The model under review builds one solid part; all positions refer to its coordinate system, in mm. A direction names the side the tool comes from. Coordinates: 2 decimals unless noted, no trailing zeros. Write each loop counter-clockwise with the first axis right and the second up, starting at its lowest first coordinate (ties: lowest second). Pieces come first, ordered by that corner, then holes.
1) For line 1 (Y direction, x = -28, z = 9); line 2 (X direction, y = -11.5, z = 5.5); line 3 (X direction, y = -22.5, z = 9.5), list the stretches that pass through material, from the lowest coordinate up.
2) Add section C-C, the plane y = -21. State the section outline as (x, z) points, then the cut area to 3 significant figures.
3) Add section A-A, the plane z = 6. State the section outline as (x, y) points.
4) For P1, Ø3, axis at y = 9, z = 7.5, coming from the +X side; P2, Ø2, axis at x = -16, y = 25.5, coming from the +Z side; P3, Ø5, axis at x = 2.5, z = 5, coming from the +Y side; P4, Ø1, axis at x = -36.5, z = 4, coming from the -Y side, all flat-tipped, find the tip position at first contact; note any pin that passes through.
5) Add section B-B, the plane x = 32. State the section outline as (y, z) points, then the cut area to 3 significant figures.
6) Mouldability with a two-part tool opening along Y and no side actions: class faces 1 (the conical face through (36.221, -23.091, 11.017)), 2 (the flat face through (0, -25.15, 7)), 3 (the flat face through (-39.3, 0.3, 2)) as released by +Y, released by -Y, zero draft, split by the parting line, or undercut.
7) Machinability: for faces 4 (the flat face through (-38.3, 0, 7)), 5 (the conical face through (-36.221, 23.091, 11.017)), 6 (the flat face through (36.3, 0, 6)), 7 (the cylindrical face through (-37.4, -24.29, 7.19)), 8 (the flat face through (0, 25.15, 7)), which of the approach directions +Z, -Z, +X, -X, +Y, -Y give a long, thin tool a straight path to every point of the face, cutting with its end or side? Answer none if there is none.
Autodesk Fusion 360 part; units mm, degrees
sketch "Sketch1" plane through (0, 0, 0) normal (0, 0, 1) x (1, 0, 0)
  line L0 (36, -22.85) -> (-36, -22.85) construction
  line L1 (-36, -22.85) -> (-36, 22.85) construction
  line L2 (-36, 22.85) -> (36, 22.85) construction
  line L3 (36, 22.85) -> (36, -22.85) construction
  line L4 (36, -22.85) -> (-36, 22.85) construction
  line L5 (-36, -22.85) -> (36, 22.85) construction
  line L6 (35.3, -23.15) -> (-35.3, -23.15)
  line L7 (-36.3, -22.15) -> (-36.3, 22.15)
  line L8 (-35.3, 23.15) -> (35.3, 23.15)
  line L9 (36.3, 22.15) -> (36.3, -22.15)
  arc A0 (-35.3, 23.15) -> (-36.3, 22.15) centre (-35.3, 22.15) ccw
  arc A1 (35.3, -23.15) -> (36.3, -22.15) centre (35.3, -22.15) ccw
  arc A2 (36.3, 22.15) -> (35.3, 23.15) centre (35.3, 22.15) ccw
  arc A3 (-36.3, -22.15) -> (-35.3, -23.15) centre (-35.3, -22.15) ccw
  arc A4 (38.3, 22.15) -> (35.3, 25.15) centre (35.3, 22.15) ccw
  line L10 (-35.3, 25.15) -> (35.3, 25.15)
  arc A5 (-35.3, 25.15) -> (-38.3, 22.15) centre (-35.3, 22.15) ccw
  line L11 (-38.3, -22.15) -> (-38.3, 22.15)
  arc A6 (-38.3, -22.15) -> (-35.3, -25.15) centre (-35.3, -22.15) ccw
  line L12 (35.3, -25.15) -> (-35.3, -25.15)
  arc A7 (35.3, -25.15) -> (38.3, -22.15) centre (35.3, -22.15) ccw
  line L13 (38.3, 22.15) -> (38.3, -22.15)
  arc A8 (46.3, 22.15) -> (35.3, 33.15) centre (35.3, 22.15) ccw
  line L14 (-35.3, 33.15) -> (35.3, 33.15)
  arc A9 (-35.3, 33.15) -> (-46.3, 22.15) centre (-35.3, 22.15) ccw
  line L15 (-46.3, -22.15) -> (-46.3, 22.15)
  arc A10 (-46.3, -22.15) -> (-35.3, -33.15) centre (-35.3, -22.15) ccw
  line L16 (35.3, -33.15) -> (-35.3, -33.15)
  arc A11 (35.3, -33.15) -> (46.3, -22.15) centre (35.3, -22.15) ccw
  line L17 (46.3, 22.15) -> (46.3, -22.15)
  dimension "d3" = 45.7
  dimension "d4" = 72
  dimension "d6" = 1
  dimension "d7" = -2
  dimension "d8" = -10
extrude "Extrude1" add sketch "Sketch1" along normal blind 11.5 contours A4 L10 A5 L11 A6 L12 A7 L13
extrude "Extrude2" add sketch "Sketch1" along normal blind 1 contours A8 L14 A9 L15 A10 L16 A11 L17
chamfer "Chamfer1" distance 0.8 angle 45 8 edges at (0, 23.15, 11.5) (36.0071, 22.8571, 11.5) (36.3, 0, 11.5) (36.0071, -22.8571, 11.5) (0, -23.15, 11.5) (-36.0071, -22.8571, 11.5) (-36.3, 0, 11.5) (-36.0071, 22.8571, 11.5)
chamfer "Chamfer2" distance 2 angle 45 8 edges at (0, 25.15, 1) (-37.4213, 24.2713, 1) (-38.3, 0, 1) (-37.4213, -24.2713, 1) (0, -25.15, 1) (37.4213, -24.2713, 1) (38.3, 0, 1) (37.4213, 24.2713, 1)
chamfer "Chamfer3" distance 0.5 angle 45 16 edges at (0, 33.15, 0) (43.0782, 29.9282, 0) (46.3, 0, 0) (43.0782, -29.9282, 0) (0, -33.15, 0) (-43.0782, -29.9282, 0) (-46.3, 0, 0) (-43.0782, 29.9282, 0) (0, 23.15, 0) (36.0071, 22.8571, 0) (36.3, 0, 0) (36.0071, -22.8571, 0) (0, -23.15, 0) (-36.0071, -22.8571, 0) (-36.3, 0, 0) (-36.0071, 22.8571, 0)
Geometry results:
1. line 1: y = -25.15 to -23.15, 23.15 to 25.15
1. line 2: x = -38.3 to -36.3, 36.3 to 38.3
1. line 3: x = -38.28 to -36.24, 36.24 to 38.28
2. outline: (-46.3, 0.5) - (-45.8, 0) - (-36.8, 0) - (-36.3, 0.5) - (-36.3, 10.7) - (-37.1, 11.5) - (-38.3, 11.5) - (-38.3, 3) - (-40.3, 1) - (-46.3, 1) - close; (36.3, 0.5) - (36.8, 0) - (45.8, 0) - (46.3, 0.5) - (46.3, 1) - (40.3, 1) - (38.3, 3) - (38.3, 11.5) - (37.1, 11.5) - (36.3, 10.7) - close
2. area: 64.9 mm2
3. outline: (-38.3, -22.15) arc R3 ccw to (-35.3, -25.15) - (35.3, -25.15) arc R3 ccw to (38.3, -22.15) - (38.3, 22.15) arc R3 ccw to (35.3, 25.15) - (-35.3, 25.15) arc R3 ccw to (-38.3, 22.15) - close; hole (-36.3, -22.15) arc R1 ccw to (-35.3, -23.15) - (35.3, -23.15) arc R1 ccw to (36.3, -22.15) - (36.3, 22.15) arc R1 ccw to (35.3, 23.15) - (-35.3, 23.15) arc R1 ccw to (-36.3, 22.15) - close
4. P1: stops at x = 38.3
4. P2: stops at z = 11.5
4. P3: stops at y = 25.65
4. P4: stops at y = -25.07
5. outline: (-33.15, 0.5) - (-32.65, 0) - (-23.65, 0) - (-23.15, 0.5) - (-23.15, 10.7) - (-23.95, 11.5) - (-25.15, 11.5) - (-25.15, 3) - (-27.15, 1) - (-33.15, 1) - close; (23.15, 0.5) - (23.65, 0) - (32.65, 0) - (33.15, 0.5) - (33.15, 1) - (27.15, 1) - (25.15, 3) - (25.15, 11.5) - (23.95, 11.5) - (23.15, 10.7) - close
5. area: 64.9 mm2
6. face 1: undercut
6. face 2: released by -Y
6. face 3: zero draft
7. face 4: +Z, -X, +Y, -Y
7. face 5: +Z
7. face 6: +Z, -Z
7. face 7: +Z, -X, -Y
7. face 8: +Z, +X, -X, +Y
